Here's how the part is built. I have some questions about the finished solid (model axes, mm). Face numbers are marked on the shaded views. Coordinates: 2 decimals unless noted, no trailing zeros. Write each loop counter-clockwise with the first axis right and the second up, starting at its lowest first coordinate (ties: lowest second). Pieces come first, ordered by that corner, then holes.
(1) For pin 1 Ø7.5 at (x, y) = (-34.75, -34.75) entering from -Z, with a flat end and sliding along its axis, tell me the tip position at first contact or that it passes through.
(2) Imagine slicing it at A-A, the plane x = 0. List the corners of the cut face in (y, z) for me (1 decimal), plus the area to 3 significant figures.
(3) Imagine slicing it at C-C, the plane x = 34.75. List the corners of the cut face in (y, z) for me (3 decimals).
(4) Imagine slicing it at B-B, the plane y = 34.75. State how many separate pieces and enclosed holes the cut face has, plus the area to 3 significant figures.
(5) Please list where these lines run through material, in increasing order: probe 1 along Y at (x, z) = (35, 11.5); probe 2 along Z at (x, y) = (-10.5, -23.5) (3 decimals); probe 3 along Y at (x, z) = (24, 2).
(6) Thinking about a two-plate mould opening in X: for the marked faces 1 and 2, which applies, released by +X, released by -X, zero draft, split by the parting line, or undercut?
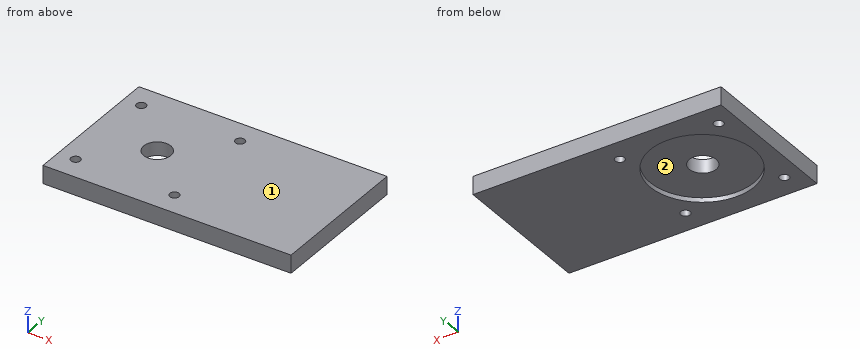
Autodesk Inventor part; units mm, degrees
ref_plane "YZ Plane" through (0, 0, 0) normal (1, 0, 0) x (0, 1, 0)
ref_plane "XZ Plane" through (0, 0, 0) normal (0, 1, 0) x (-1, 0, 0)
ref_plane "XY Plane" through (0, 0, 0) normal (0, 0, 1) x (1, 0, 0)
sketch "Sketch1" plane through (0, 0, 0) normal (0, 0, 1) x (1, 0, 0)
  line L0 (-42.925, -19.7) -> (-38.525, -19.7)
  arc A0 (-38.525, -28.9) -> (-38.525, -19.7) centre (-38.525, -24.3) ccw
  line L1 (-38.525, -28.9) -> (-42.925, -28.9)
  line L2 (-42.925, -37.425) -> (-42.925, -28.9)
  arc A1 (-42.925, -37.425) -> (-37.425, -42.925) centre (-37.425, -37.425) ccw
  line L3 (19.7, -42.925) -> (-37.425, -42.925)
  line L4 (19.7, -42.925) -> (19.7, -38.525)
  arc A2 (28.9, -38.525) -> (19.7, -38.525) centre (24.3, -38.525) ccw
  line L5 (28.9, -38.525) -> (28.9, -42.925)
  line L6 (37.425, -42.925) -> (28.9, -42.925)
  arc A3 (37.425, -42.925) -> (42.925, -37.425) centre (37.425, -37.425) ccw
  line L7 (42.925, 19.7) -> (42.925, -37.425)
  line L8 (42.925, 19.7) -> (38.525, 19.7)
  arc A4 (38.525, 28.9) -> (38.525, 19.7) centre (38.525, 24.3) ccw
  line L9 (38.525, 28.9) -> (42.925, 28.9)
  line L10 (42.925, 37.425) -> (42.925, 28.9)
  arc A5 (42.925, 37.425) -> (37.425, 42.925) centre (37.425, 37.425) ccw
  line L11 (-19.7, 42.925) -> (37.425, 42.925)
  line L12 (-19.7, 42.925) -> (-19.7, 38.525)
  arc A6 (-28.9, 38.525) -> (-19.7, 38.525) centre (-24.3, 38.525) ccw
  line L13 (-28.9, 38.525) -> (-28.9, 42.925)
  line L14 (-37.425, 42.925) -> (-28.9, 42.925)
  arc A7 (-37.425, 42.925) -> (-42.925, 37.425) centre (-37.425, 37.425) ccw
  line L15 (-42.925, -19.7) -> (-42.925, 37.425)
  circle A8 centre (34.75, -34.75) radius 3.3
  circle A9 centre (-34.75, -34.75) radius 3.3
  circle A10 centre (34.75, 34.75) radius 3.3
  circle A11 centre (-34.75, 34.75) radius 3.3
  circle A12 centre (0, 0) radius 36.5125
  line L16 (127.3875, 50.7471) -> (127.3875, -50.8529)
  line L17 (127.3875, 50.7471) -> (-47.0237, 50.7471)
  line L18 (-47.0237, 50.7471) -> (-47.0237, -50.8529)
  line L19 (-47.0237, -50.8529) -> (127.3875, -50.8529)
  point P0 (0, 0)
  dimension "d0" = 101.6
extrude "Extrusion1" add sketch "Sketch1" along normal blind 12.7 contours L15 A7 L14 L13 A6 L12 L11 A5 L10 L9 A4 L8 L7 A3 L6 L5 A2 L4 L3 A1 L2 L1 A0 L0 | L16 L19 L18 L17
sketch "Sketch2" plane through (0, 0, 12.7) normal (0, 0, 1) x (1, 0, 0)
  line L0 (127.3875, -50.8529) -> (127.3875, 50.7471)
  line L1 (127.3875, 50.7471) -> (-47.0237, 50.7471)
  line L2 (-47.0237, 50.7471) -> (-47.0237, -50.8529)
  line L3 (-47.0237, -50.8529) -> (127.3875, -50.8529)
  circle A0 centre (0, 0) radius 36.5125
  circle A1 centre (34.75, -34.75) radius 3.3
  circle A2 centre (-34.75, 34.75) radius 3.3
  circle A3 centre (34.75, 34.75) radius 3.3
  circle A4 centre (-34.75, -34.75) radius 3.3
  circle A5 centre (0, -0.6853) radius 9.525
  point P0 (0, 0)
  dimension "d3" = 19.05
extrude "Extrusion2" add sketch "Sketch2" against normal blind 9.525 contours A0
properties part number "Stepper Plate"
Recorded:
1. pin 1: stops at z = 0
2. outline: (-50.9, 0) - (-36.5, 0) - (-36.5, 3.2) - (-10.2, 3.2) - (-10.2, 12.7) - (-50.9, 12.7) - close; (8.8, 3.2) - (36.5, 3.2) - (36.5, 0) - (50.7, 0) - (50.7, 12.7) - (8.8, 12.7) - close
2. area: 877 mm2
3. outline: (-50.853, 0) - (-38.05, 0) - (-38.05, 12.7) - (-50.853, 12.7) - close; (-31.45, 0) - (-11.207, 0) - (-11.207, 3.175) - (11.207, 3.175) - (11.207, 0) - (31.45, 0) - (31.45, 12.7) - (-31.45, 12.7) - close; (38.05, 0) - (50.747, 0) - (50.747, 12.7) - (38.05, 12.7) - close
4. separate pieces: 3
4. enclosed holes: 0
4. area: 1,980 mm2
5. probe 1: y = -50.85 to -38.04, -31.46 to 31.46, 38.04 to 50.75
5. probe 2: z = 3.175 to 12.7
5. probe 3: y = -50.85 to -27.52, 27.52 to 50.75
6. face 1: zero draft
6. face 2: undercut
